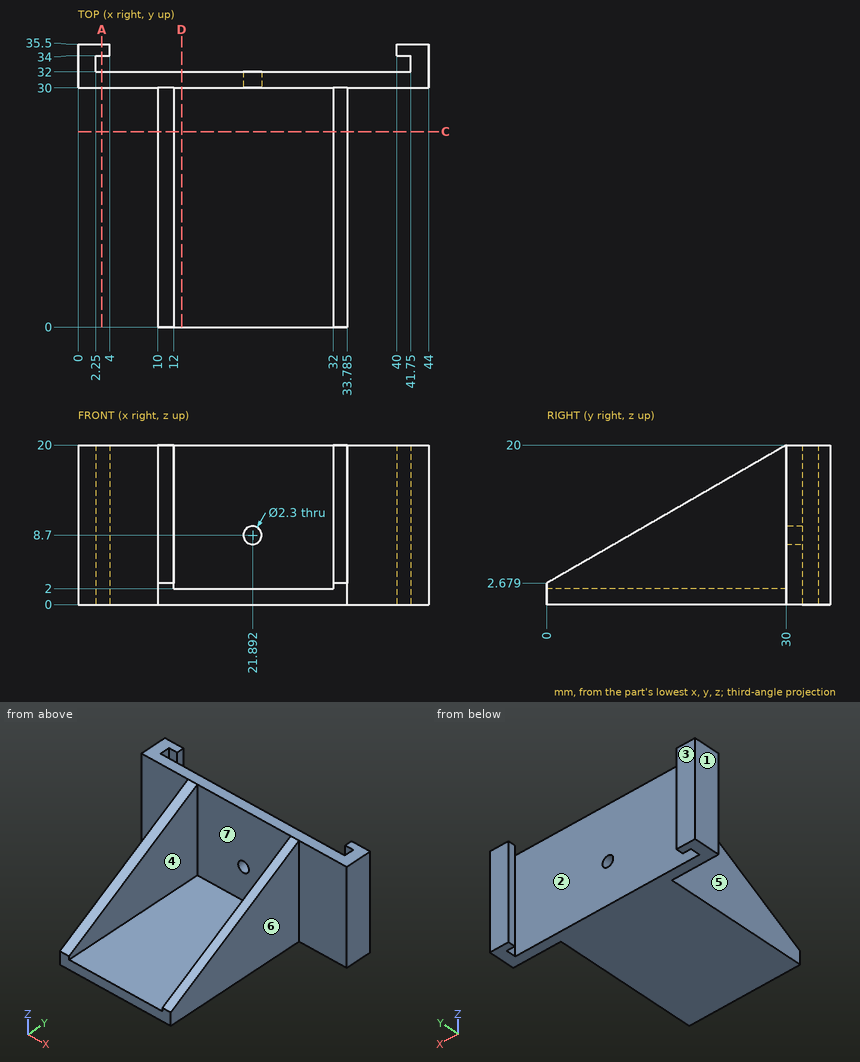
Source: three-view drawing plus pictorial views. Frame: mm from the lowest corner of the part. A direction names the side the tool comes from. Coordinates: 2 decimals unless noted, no trailing zeros. Loops run counter-clockwise (first coordinate to the right, second up) from the corner with the lowest first, then second, coordinate; pieces in that order, holes last. Notation, with made-up numbers: (-37.75, 82.5) - (-28.75, 82.5) arc R18 cw to (-28.75, 112.5) - close; hole circle Ø1 at (-9.5, 2.25). An arc over 180 degrees is marked (long way). Answer in a Markdown table with one row per item. Add a question column.
Item 1: Line query: line 1 along Y through (x, z) = (41, 13.25); line 2 along X through (y, z) = (31.4, 8.7); line 3 along X through (y, z) = (14, 10.5) (1 decimal). Output: solid intervals per line, ascending. Write a range as [from, to].
Item 2: Access query for the marked faces 5, 6 and 7. Directions: +Z, -Z, +X, -X, +Y, -Y. A direction counts if a zero-diameter tool reaches every point of the face in a straight line with its end or side. Return the directions, or none.
Item 3: Section query C-C on y = 24.5. Return the cut outline in (x, z) (1 decimal).
Item 4: Section query A-A on x = 3. Return the cut outline in (y, z).
Item 5: Section query D-D on x = 13. Return the cut outline in (y, z).
Item 6: Contact query for flat-ended pins moving along their axis: P1, Ø0.9, axis at x = 40.5, z = 10.5, coming from the -Y side; P2, Ø10, axis at y = 13.5, z = 9, coming from the -X side; P3, Ø1.5, axis at x = 11.5, y = 16, coming from the +Z side; P4, Ø4, axis at x = 6.5, y = 19, coming from the -Z side. Output: stop coordinate, or through.
Item 7: Mould query, pull axis X, two halves, no side actions, for the marked faces 1, 2, 3 and 4. Classes: released by +X, released by -X, zero draft, split by the parting line, or undercut.
Recorded:
| question | item | result |
|---|---|---|
| 1 | line 1 | [30, 32], [34, 35.5] |
| 1 | line 2 | [0, 20.74], [23.04, 44] |
| 1 | line 3 | [10, 12], [32, 33.8] |
| 2 | face 5 | +Z, -Z, -X, -Y |
| 2 | face 6 | +Z, -Z, +X, -Y |
| 2 | face 7 | +Z, -Y |
| 3 | outline | (10, 0) - (33.8, 0) - (33.8, 16.8) - (32, 16.8) - (32, 2) - (12, 2) - (12, 16.8) - (10, 16.8) - close |
| 4 | outline | (30, 0) - (32, 0) - (32, 20) - (30, 20) - close; (34, 0) - (35.5, 0) - (35.5, 20) - (34, 20) - close |
| 5 | outline | (0, 0) - (32, 0) - (32, 20) - (30, 20) - (30, 2) - (0, 2) - close |
| 6 | P1 | y = 30 |
| 6 | P2 | x = 10 |
| 6 | P3 | z = 12.35 |
| 6 | P4 | through |
| 7 | face 1 | released by -X |
| 7 | face 2 | undercut |
| 7 | face 3 | zero draft |
| 7 | face 4 | undercut |
